CAD build for the part. Positions are in the model's coordinates, mm. Give positions to 0.01 mm unless a question says otherwise; leave off trailing zeros. Write each loop counter-clockwise with the first axis right and the second up, starting at its lowest first coordinate (ties: lowest second). Pieces come first, ordered by that corner, then holes. Notation, with made-up numbers: (14.25, 0) -> (45.25, 0) arc R21 cw to (45.25, 34) -> close; hole circle Ø1 at (72.25, 47.25). An arc over 180 degrees is marked (long way). Answer as a JSON object with one key per item and string values.
```python
from build123d import *

# Parameters (mm, degrees)
CROQUIS1_R              = 4
SALIENTE_EXTRUIR1_DEPTH = 46
CROQUIS2_W              = 20
CROQUIS2_H              = 8
SALIENTE_EXTRUIR2_DEPTH = 5
CORTAR_EXTRUIR1_REACH   = 54.125
CROQUIS3_R              = 1.5
CROQUIS4_R              = 1.5
CORTAR_EXTRUIR2_DEPTH   = 5


with BuildPart() as part:
    # Croquis1 → Saliente-Extruir1 (new body)
    with BuildSketch(Plane(origin=(0, 0, 0), x_dir=(0, 1, 0), z_dir=(0, 0, 1))):
        with Locations(Location((0, 0, 0), (0, 0, 270))):
            Circle(CROQUIS1_R)
    extrude(amount=SALIENTE_EXTRUIR1_DEPTH)

    # Croquis2 → Saliente-Extruir2 (add)
    with BuildSketch(Plane.XY.offset(46)):
        Rectangle(CROQUIS2_W, CROQUIS2_H)
    extrude(amount=SALIENTE_EXTRUIR2_DEPTH)

    # Croquis3 → Cortar-Extruir1 (cut, up to next)
    with BuildSketch(Plane.XY.offset(51), mode=Mode.PRIVATE) as cortar_extruir1_sk1:
        with Locations((6, 0)):
            Circle(CROQUIS3_R)
    cortar_extruir1_tool1 = extrude(cortar_extruir1_sk1.sketch, amount=-CORTAR_EXTRUIR1_REACH, mode=Mode.PRIVATE) & part.part
    # Croquis3 → Cortar-Extruir1 (cut, up to next)
    with BuildSketch(Plane.XY.offset(51), mode=Mode.PRIVATE) as cortar_extruir1_sk2:
        with Locations(Location((-6, 0, 0), (0, 0, 180))):
            Circle(CROQUIS3_R)
    cortar_extruir1_tool2 = extrude(cortar_extruir1_sk2.sketch, amount=-CORTAR_EXTRUIR1_REACH, mode=Mode.PRIVATE) & part.part
    add(cortar_extruir1_tool1.solids().sort_by_distance((6, 0, 51))[0], mode=Mode.SUBTRACT)
    add(cortar_extruir1_tool2.solids().sort_by_distance((-6, 0, 51))[0], mode=Mode.SUBTRACT)

    # Croquis4 → Cortar-Extruir2 (cut, symmetric)
    with BuildSketch(Plane(origin=(0, 0, 0), x_dir=(-1, 0, 0), z_dir=(0, 1, 0))):
        with Locations(Location((0, 20.5, 0), (0, 0, 90))):
            Circle(CROQUIS4_R)
    extrude(amount=CORTAR_EXTRUIR2_DEPTH, both=True, mode=Mode.SUBTRACT)


solid = part.part
```
1) Slice it at D-D (x = -8). List the corners of the cut face in (y, z).
Model answer:
{"outline": "(-4, 46) -> (4, 46) -> (4, 51) -> (-4, 51) -> close"}
2) Slice it at B-B (y = 3). List the corners of the cut face in (x, z).
Model answer:
{"outline": "(-10, 46) -> (-2.65, 46) -> (-2.65, 0) -> (2.65, 0) -> (2.65, 46) -> (10, 46) -> (10, 51) -> (-10, 51) -> close; hole circle Ø3 at (0, 20.5)"}
3) Slice it at C-C (z = 20.5). List the corners of the cut face in (x, y).
Model answer:
{"outline": "(-1.5, -3.71) -> (-1.5, 3.71) arc R4 ccw to start; (1.5, -3.71) arc R4 ccw to (1.5, 3.71) -> close"}
4) Mould opens along Z. For faces 1 (the flat face through (0, 0, 51)), 2 (the cylindrical face through (0, 0, 19)), 3 (the flat face through (8, 0, 46)), 4 (the cylindrical face through (-0.867, -3.905, 22.678)) say: released by +Z, released by -Z, zero draft, split by the parting line, or undercut.
Model answer:
{"face 1": "released by +Z", "face 2": "undercut", "face 3": "released by -Z", "face 4": "zero draft"}
5) Pin check, flat tips, straight feed: pin 1 (1.5 mm diameter, centred on y = -2.5, z = 32.5, fed in from +X); pin 2 (4 mm diameter, centred on x = -7, y = 1.5, fed in from -Z); pin 3 (3.5 mm diameter, centred on x = 0, z = 20.5, fed in from +Y); pin 4 (2.5 mm diameter, centred on x = -6, y = 0, fed in from +Z). Stop position of each tip, or through.
Model answer:
{"pin 1": "stops at x = 3.6", "pin 2": "stops at z = 46", "pin 3": "stops at y = 4", "pin 4": "passes through"}
6) Slice it at A-A (x = 6). List the corners of the cut face in (y, z), then the cut area to 3 significant figures.
Model answer:
{"outline": "(-4, 46) -> (-1.5, 46) -> (-1.5, 51) -> (-4, 51) -> close; (1.5, 46) -> (4, 46) -> (4, 51) -> (1.5, 51) -> close", "area": "25.0 mm2"}
7) Wall check: probe 1 along Y at (x, z) = (-6, 47.9); probe 2 along Z at (x, y) = (5.5, 1.5); probe 3 along X at (y, z) = (2, 20.5). Give the ranges that are in metal, low to high.
Model answer:
{"probe 1": "y = -4 to -1.5, 1.5 to 4", "probe 2": "z = 46 to 51", "probe 3": "x = -3.46 to -1.5, 1.5 to 3.46"}
